```python
from build123d import *

# Parameters (mm, degrees)
BOSS_EXTRUDE1_DEPTH = 1.5
SKETCH2_W           = 3
SKETCH2_H           = 10
CUT_EXTRUDE1_DEPTH  = 56.865910894
SKETCH3_W           = 55
SKETCH3_H           = 25
CUT_EXTRUDE2_DEPTH  = 56.865910894
CUT_EXTRUDE3_DEPTH  = 56.865910894
SKETCH7_W           = 25.2
SKETCH7_H           = 3.2
CUT_EXTRUDE6_DEPTH  = 56.865910894


with BuildPart() as part:
    # Sketch1 → Boss-Extrude1 (new, symmetric)
    with BuildSketch(Plane.XY):
        Polygon((-20, -11), (20, -11), (20, -14), (35, -14), (35, -11), (54, -11), (54, 11), (-54, 11), (-54, -11), (-35, -11), (-35, -14), (-20, -14), align=None)
    extrude(amount=BOSS_EXTRUDE1_DEPTH, both=True)

    # Sketch2 → Cut-Extrude1 (cut, through all)
    with BuildSketch(Plane.XY.offset(1.5)):
        with Locations((2.5, 0)):
            Rectangle(SKETCH2_W, SKETCH2_H)
        with Locations((52.5, 0)):
            Rectangle(SKETCH2_W, SKETCH2_H)
    extrude(amount=-CUT_EXTRUDE1_DEPTH, mode=Mode.SUBTRACT)

    # Sketch3 → Cut-Extrude2 (cut, through all)
    with BuildSketch(Plane.XY.offset(1.5)):
        with Locations((-26.5, -1.5)):
            Rectangle(SKETCH3_W, SKETCH3_H)
    extrude(amount=-CUT_EXTRUDE2_DEPTH, mode=Mode.SUBTRACT)

    # Sketch4 → Cut-Extrude3 (cut, through all)
    with BuildSketch(Plane(origin=(0, 0, -1.5), x_dir=(-1, 0, 0), z_dir=(0, 0, -1))):
        with BuildLine():
            Line((-7, -11), (-7, -9))
            ThreePointArc((-7, -9), (-7.585786438, -7.585786438), (-9, -7))
            Line((-9, -7), (-13, -7))
            ThreePointArc((-13, -7), (-14.414213562, -7.585786438), (-15, -9))
            Line((-15, -9), (-15, -11))
            Line((-15, -11), (-7, -11))
        make_face()
    extrude(amount=-CUT_EXTRUDE3_DEPTH, mode=Mode.SUBTRACT)

    # Sketch7 → Cut-Extrude6 (cut, through all)
    with BuildSketch(Plane.XY.offset(1.5)):
        with Locations((27.5, 9.4)):
            Rectangle(SKETCH7_W, SKETCH7_H)
    extrude(amount=-CUT_EXTRUDE6_DEPTH, mode=Mode.SUBTRACT)


solid = part.part
```
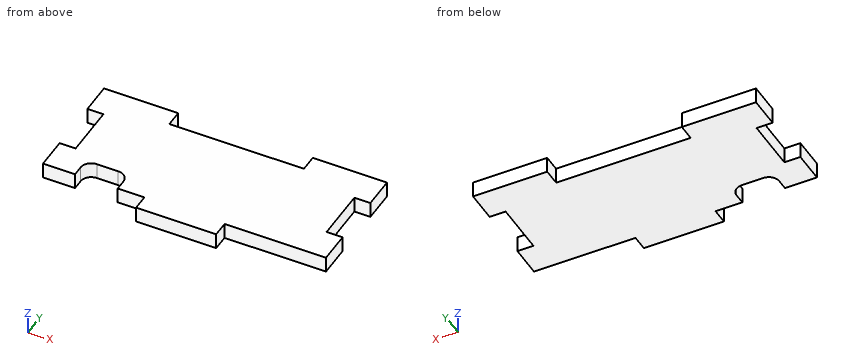
Can you work these out from the model? Positions are in its coordinate system, mm. Give positions to 0.01 mm unless a question says otherwise; leave off trailing zeros. Order: outer loops, then holes, each group sorted by start corner. A loop starts at its lowest first (then second) coordinate and runs counter-clockwise, first axis right, second up. Notation, with made-up numbers: (9, 44) - (23, 44) arc R24 cw to (23, 68) - close; hole circle Ø6 at (4.5, 54.5). An arc over 180 degrees is marked (long way). Use a Markdown table: item, result. Add a question column.
Q1. If we section it at A-A on y = 8.5: Write out the boundary of the cut face in (x, z).
Q2. Please list where these lines run through material, in increasing order: line 1 along Y through (x, z) = (51.5, -0.3); line 2 along X through (y, z) = (8.25, -0.75); line 3 along X through (y, z) = (-4.5, -0.75).
Q3. I'm going to push flat-ended pins straight in: pin 1 (1 mm diameter, centred on x = 24, z = -0.5, fed in from +Y); pin 2 (0.9 mm diameter, centred on x = 44, z = 0.5, fed in from -Y); pin 3 (1.5 mm diameter, centred on y = -1, z = 0.5, fed in from -X). Where does each tip first touch, or does it pass through?
Q4. If we section it at C-C on y = -10.5: Write out the boundary of the cut face in (x, z).
Q5. If we section it at B-B on z = 0.3: Write out the boundary of the cut face in (x, y), plus the area to 3 significant figures.
Q6. If we section it at D-D on x = 39: Write out the boundary of the cut face in (y, z), plus the area to 3 significant figures.
Answers follow:
| question | item | result |
|---|---|---|
| 1 | outline | (1, -1.5) - (14.9, -1.5) - (14.9, 1.5) - (1, 1.5) - close; (40.1, -1.5) - (54, -1.5) - (54, 1.5) - (40.1, 1.5) - close |
| 2 | line 1 | y = -11 to -5, 5 to 11 |
| 2 | line 2 | x = 1 to 14.9, 40.1 to 54 |
| 2 | line 3 | x = 4 to 51 |
| 3 | pin 1 | stops at y = 7.8 |
| 3 | pin 2 | stops at y = -11 |
| 3 | pin 3 | stops at x = 4 |
| 4 | outline | (1, -1.5) - (7, -1.5) - (7, 1.5) - (1, 1.5) - close; (15, -1.5) - (54, -1.5) - (54, 1.5) - (15, 1.5) - close |
| 5 | outline | (1, -11) - (7, -11) - (7, -9) arc R2 cw to (9, -7) - (13, -7) arc R2 cw to (15, -9) - (15, -11) - (20, -11) - (20, -14) - (35, -14) - (35, -11) - (54, -11) - (54, -5) - (51, -5) - (51, 5) - (54, 5) - (54, 11) - (40.1, 11) - (40.1, 7.8) - (14.9, 7.8) - (14.9, 11) - (1, 11) - (1, 5) - (4, 5) - (4, -5) - (1, -5) - close |
| 5 | area | 1,040 mm^2 |
| 6 | outline | (-11, -1.5) - (7.8, -1.5) - (7.8, 1.5) - (-11, 1.5) - close |
| 6 | area | 56.4 mm^2 |
